```python
from build123d import *
from build123d.topology import SkipClean

# Parameters (mm, degrees)
SKETCH1_R           = 2.159
BOSS_EXTRUDE1_DEPTH = 3.175
SKETCH3_R           = 4.7625
SKETCH3_R_2         = 2.159
BOSS_EXTRUDE2_DEPTH = 4.7625


with BuildPart() as part:
    # Sketch1 → Boss-Extrude1 (new, symmetric)
    with BuildSketch(Plane.XY):
        with BuildLine():
            Line((0, -4.7625), (-12.7, -4.7625))
            ThreePointArc((-12.7, -4.7625), (-15.733752874, -3.67120549), (-17.377178039, -0.897447401))
            Line((-17.377178039, -0.897447401), (-20.392626251, 14.818000811))
            ThreePointArc((-20.392626251, 14.818000811), (-17.946232861, 19.923179917), (-12.347852166, 19.083044257))
            Line((-12.347852166, 19.083044257), (3.367596045, 3.367596045))
            ThreePointArc((3.367596045, 3.367596045), (4.399976274, -1.822529847), (0, -4.7625))
        make_face()
        with Locations((-12.7, 0)):
            Circle(SKETCH1_R, mode=Mode.SUBTRACT)
        with Locations((-15.715448212, 15.715448212)):
            Circle(SKETCH1_R, mode=Mode.SUBTRACT)
        Circle(SKETCH1_R, mode=Mode.SUBTRACT)
    extrude(amount=BOSS_EXTRUDE1_DEPTH, both=True)

    # Sketch3 → Boss-Extrude2 (add, symmetric)
    with SkipClean():  # the faces are left unmerged after this step: merging them gives an invalid solid
        with BuildSketch(Plane.XY.offset(3.175)):
            with Locations(Location((0, 0, 0), (0, 0, 270))):
                Circle(SKETCH3_R)
            Circle(SKETCH3_R_2, mode=Mode.SUBTRACT)
        extrude(amount=BOSS_EXTRUDE2_DEPTH, both=True)


solid = part.part
```
CAD build for the part. Positions are in the model's coordinates, mm. Give positions to 0.01 mm unless a question says otherwise; leave off trailing zeros. Write each loop counter-clockwise with the first axis right and the second up, starting at its lowest first coordinate (ties: lowest second). Pieces come first, ordered by that corner, then holes. Notation, with made-up numbers: M -37.75,-30 L -6.75,-30 A21 cw -6.75,-12 Z; hole C 49.25,-39.75 d4. An arc over 180 degrees is marked long. Return JSON: item names as keys, results as strings. Group by question number.
(1) Band-saw the part on B-B (x = -16.75). Give the cut face in (y, z) (3 decimals).
(2) Drill centre lines: L1, parallel to Y at x = -16.5, z = -0.25; L2, parallel to Z at x = -1, y = 6.75 (3 decimals); L3, parallel to Y at x = -12.7, z = 1. Where is each one in solid material? Low to high. Write a range as [from, to].
(3) Band-saw the part on C-C (z = -2.5). Give the cut face in (x, y) (1 decimal), and give its area (3 significant figures).
(4) Band-saw the part on D-D (z = 6.25). Give the cut face in (x, y) (1 decimal), and give its area (3 significant figures).
(5) Flat gauge pins, fed straight in: pin 1 Ø6 at (x, z) = (-12.5, -1.5) entering from +Y; pin 2 Ø5 at (x, y) = (-8, 10) entering from +Z (3 decimals); pin 3 Ø1 at (y, z) = (16, 0.5) entering from +X; pin 4 Ø5 at (x, y) = (0, 0) entering from -Z (3 decimals). Where does each tip first touch, or does it go through?
(6) Band-saw the part on A-A (y = -0.5). Give the cut face in (x, z) (1 decimal).
(7) Mould opens along Y. For faces 1 (the face through (-16.183, 13.608, -0.044)), 2 (the face through (-4.6, 11.335, 0.044)), 3 (the face through (1.13, -2.05, 7.938)) say: pulls with the +Y half, pulls with the -Y half, needs draft (parallel to the pull), parting line crosses it, or undercut.
Entries:
{
 "1": {"outline": "M -2.506,-3.175 L 13.82,-3.175 L 13.82,3.175 L -2.506,3.175 Z; M 17.61,-3.175 L 20.364,-3.175 L 20.364,3.175 L 17.61,3.175 Z"},
 "2": {"L1": "y = [-2.87, 13.7], [17.73, 20.41]", "L2": "z = [-3.175, 3.175]", "L3": "y = [-4.76, -2.16], [2.16, 19.4]"},
 "3": {"outline": "M -20.4,14.8 L -17.4,-0.9 A4.8 ccw -12.7,-4.8 L 0,-4.8 A4.8 ccw 3.4,3.4 L -12.3,19.1 A4.8 ccw Z; hole C -15.7,15.7 d4.3; hole C -12.7,0 d4.3; hole C 0,0 d4.3", "area": "370 mm^2"},
 "4": {"outline": "C 0,0 d9.5; hole C 0,0 d4.3", "area": "56.6 mm^2"},
 "5": {"pin 1": "stops at y = 20.47", "pin 2": "stops at z = 3.175", "pin 3": "stops at x = -8.76", "pin 4": "stops at z = -3.175"},
 "6": {"outline": "M -17.5,-3.2 L -14.8,-3.2 L -14.8,3.2 L -17.5,3.2 Z; M -10.6,-3.2 L -2.1,-3.2 L -2.1,7.9 L -4.7,7.9 L -4.7,3.2 L -10.6,3.2 Z; M 2.1,-3.2 L 4.7,-3.2 L 4.7,7.9 L 2.1,7.9 Z"},
 "7": {"face 1": "undercut", "face 2": "pulls with the +Y half", "face 3": "needs draft"}
}
